For this review, take the finished solid that the model builds, in its own axes (mm). A direction names the side the tool comes from. Give positions to 0.01 mm unless a question says otherwise; leave off trailing zeros. Order: outer loops, then holes, each group sorted by start corner. A loop starts at its lowest first (then second) coordinate and runs counter-clockwise, first axis right, second up. Notation, with made-up numbers: (71.5, 12.5) - (85.5, 12.5) arc R19 ccw to (85.5, 44.5) - close; hole circle Ø7 at (-1.5, 52.5). An arc over 180 degrees is marked (long way). Use a Markdown table: item, result. Add a question column.
1) Clearance check with flat-ended pins moving along their axes: P1, Ø2, axis at x = -1, y = -1, coming from the -Z side; P2, Ø1, axis at y = 2.5, z = 4.5, coming from the -X side; P3, Ø1.7, axis at x = 0, y = 0, coming from the +Z side; P4, Ø1, axis at x = -1, z = 12.5, coming from the -Y side. State where each tip first meets the part, or that it passes through.
2) Mouldability with a two-part tool opening along Y and no side actions: class faces 1 (the face through (-0.1, -2.4, 0)), 2 (the face through (1.79, 1.8, 6.24)), 3 (the face through (-0.809, -3.645, 6.843)) as released by +Y, released by -Y, zero draft, split by the parting line, or undercut.
3) We need section A-A on z = 9. Write out the cut boundary in (x, y), then the cut area to 3 significant figures.
4) We need section B-B on x = 0. Write out the cut boundary in (y, z), then the cut area to 3 significant figures.
5) Machinability: for faces 4 (the face through (-0.49, -2.207, 15.903)), 5 (the face through (1, 1, 17.983)), 6 (the face through (1.8, -1.79, 6.24)), which of the approach directions +Z, -Z, +X, -X, +Y, -Y give a long, thin tool a straight path to every point of the face, cutting with its end or side? Answer none if there is none.
6) We need section D-D on x = 1.5. Write out the cut boundary in (y, z), then the cut area to 3 significant figures.
7) Wall thickness on L1, parallel to Y at x = 0, z = 15; L2, parallel to Z at x = -0.75, y = -3.5; L3, parallel to Z at x = -0.75, y = -1.75: over which ranges is each line inside the solid? List them lowest first.
```python
from build123d import *

# Parameters (mm, degrees)
F0_R     = 3.7338
F1_DEPTH = 13.8811
F2_R     = 2.2606
F3_DEPTH = 4.1021
F4_R     = 1.0414
F5_DEPTH = 47.0154
F6_R     = 2.53873
F7_DEPTH = 12.6492
F8_R     = 3.7338
F9_DEPTH = 13.5382


with BuildPart() as f1:
    # F0 (on Top) → F1 (new body)
    with BuildSketch(Plane.XY):
        Circle(F0_R)
    extrude(amount=F1_DEPTH)

    # F2 (on face) → F3 (join)
    with BuildSketch(Plane.XY.offset(13.8811)):
        Circle(F2_R)
    extrude(amount=F3_DEPTH)

    # F4 (on face) → F5 (cut)
    with BuildSketch(Plane.XY.offset(17.9832)):
        Circle(F4_R)
    extrude(amount=-F5_DEPTH, mode=Mode.SUBTRACT)

    # F6 (on face) → F7 (cut)
    with BuildSketch(Plane(origin=(0, 0, 0), x_dir=(1, 0, 0), z_dir=(0, 0, -1))):
        Circle(F6_R)
    extrude(amount=-F7_DEPTH, mode=Mode.SUBTRACT)

    # F8 (on face) → F9 (join)
    with BuildSketch(Plane(origin=(0, 0, 0), x_dir=(1, 0, 0), z_dir=(0, 0, -1))):
        Circle(F8_R)
        with BuildLine():
            Line((1.1798710111, 2.2479), (2.2479, 2.2479))
            Line((2.2479, 2.2479), (2.2479, 1.1798710111))
            ThreePointArc((2.2479, 1.1798710111), (2.4649504234, 0.6075931393), (2.53873, 0))
            ThreePointArc((2.53873, 0), (2.4649504234, -0.6075931393), (2.2479, -1.1798710111))
            Line((2.2479, -1.1798710111), (2.2479, -2.2479))
            Line((2.2479, -2.2479), (1.1798710111, -2.2479))
            ThreePointArc((1.1798710111, -2.2479), (0, -2.53873), (-1.1798710111, -2.2479))
            Line((-1.1798710111, -2.2479), (-2.2479, -2.2479))
            Line((-2.2479, -2.2479), (-2.2479, -1.1798710111))
            ThreePointArc((-2.2479, -1.1798710111), (-2.53873, 0), (-2.2479, 1.1798710111))
            Line((-2.2479, 1.1798710111), (-2.2479, 2.2479))
            Line((-2.2479, 2.2479), (-1.1798710111, 2.2479))
            ThreePointArc((-1.1798710111, 2.2479), (0, 2.53873), (1.1798710111, 2.2479))
        make_face(mode=Mode.SUBTRACT)
        with BuildLine():
            Line((-1.1798710111, 2.2479), (1.1798710111, 2.2479))
            ThreePointArc((1.1798710111, 2.2479), (0, 2.53873), (-1.1798710111, 2.2479))
        make_face()
        with BuildLine():
            ThreePointArc((2.53873, 0), (2.4649504234, 0.6075931393), (2.2479, 1.1798710111))
            Line((2.2479, 1.1798710111), (2.2479, -1.1798710111))
            ThreePointArc((2.2479, -1.1798710111), (2.4649504234, -0.6075931393), (2.53873, 0))
        make_face()
        with BuildLine():
            Line((-2.2479, -1.1798710111), (-2.2479, 1.1798710111))
            ThreePointArc((-2.2479, 1.1798710111), (-2.53873, 0), (-2.2479, -1.1798710111))
        make_face()
        with BuildLine():
            ThreePointArc((-1.1798710111, -2.2479), (0, -2.53873), (1.1798710111, -2.2479))
            Line((1.1798710111, -2.2479), (-1.1798710111, -2.2479))
        make_face()
    extrude(amount=-F9_DEPTH)


solid = f1.part
```
Checked values:
| question | item | result |
|---|---|---|
| 1 | P1 | z = 12.65 |
| 1 | P2 | x = -3.15 |
| 1 | P3 | through |
| 1 | P4 | y = -3.7 |
| 2 | face 1 | zero draft |
| 2 | face 2 | undercut |
| 2 | face 3 | split by the parting line |
| 3 | outline | circle Ø7.47 at (0, 0); hole (-2.25, -1.18) arc R2.54 ccw to (-1.18, -2.25) - (1.18, -2.25) arc R2.54 ccw to (2.25, -1.18) - (2.25, 1.18) arc R2.54 ccw to (1.18, 2.25) - (-1.18, 2.25) arc R2.54 ccw to (-2.25, 1.18) - close |
| 3 | area | 25.4 mm² |
| 4 | outline | (-3.73, 0) - (-2.25, 0) - (-2.25, 12.65) - (-1.04, 12.65) - (-1.04, 17.98) - (-2.26, 17.98) - (-2.26, 13.88) - (-3.73, 13.88) - close; (1.04, 12.65) - (2.25, 12.65) - (2.25, 0) - (3.73, 0) - (3.73, 13.88) - (2.26, 13.88) - (2.26, 17.98) - (1.04, 17.98) - close |
| 4 | area | 54.2 mm² |
| 5 | face 4 | +Z |
| 5 | face 5 | +Z, +X, -X, +Y, -Y |
| 5 | face 6 | -Z |
| 6 | outline | (-3.42, 0) - (-2.05, 0) - (-2.05, 12.65) - (2.05, 12.65) - (2.05, 0) - (3.42, 0) - (3.42, 13.88) - (1.69, 13.88) - (1.69, 17.98) - (-1.69, 17.98) - (-1.69, 13.88) - (-3.42, 13.88) - close |
| 6 | area | 57.0 mm² |
| 7 | L1 | -2.26 to -1.04, 1.04 to 2.26 |
| 7 | L2 | 0 to 13.88 |
| 7 | L3 | 12.65 to 17.98 |
